Work out the finished part from the listing and answer in its coordinate system (mm). Coordinates: 2 decimals unless noted, no trailing zeros. Order: outer loops, then holes, each group sorted by start corner. A loop starts at its lowest first (then second) coordinate and runs counter-clockwise, first axis right, second up.
1. The part is cut by section A-A, the plane z = 85. Give the vertices of the cut face in (x, y).
2. The part is cut by section C-C, the plane x = 70. Give the vertices of the cut face in (y, z), then the cut area to 3 significant figures.
3. A flat-ended cylindrical pin translates along its axis: pin 1 Ø12.5 at (x, z) = (-45, 60) entering from +Y. Find the tip coordinate at first contact, or state that the pin passes through.
4. The part is cut by section D-D, the plane y = -3.5. Count the separate pieces of the cut face and the enclosed holes in it, then the cut area to 3 significant figures.
5. The part is cut by section B-B, the plane x = 0. Give the vertices of the cut face in (y, z), then the cut area to 3 significant figures.
6. Determine the mould class of faces 1 (the flat face through (-3, -5, 130)), 2 (the cylindrical face through (44.09, -4.93, 66.94)), 3 (the flat face through (180, -5, -2)), 4 (the flat face through (-180, -5, -2)) for opening direction X: +X half, -X half, draft (parallel to the pull), parting line (faces both ways), or undercut.
7. Find the intervals of material crossed by probe 1 along Z at (x, y) = (70, -3); probe 2 along X at (y, z) = (-1.25, -86); probe 3 along X at (y, z) = (-6.25, 81.5), in increasing order.
```python
from build123d import *

# Parameters (mm, degrees)
F0_W     = 360
F0_H     = 260
F0_R     = 20
F0_R_2   = 7
F0_R_3   = 47.5
F1_DEPTH = 10


with BuildPart() as f1:
    # F0 (on Front) → F1 (new body)
    with BuildSketch(Plane.XZ):
        Rectangle(F0_W, F0_H)
        with Locations((-70, -85)):
            Circle(F0_R, mode=Mode.SUBTRACT)
        with Locations((-45, -60)):
            Circle(F0_R_2, mode=Mode.SUBTRACT)
        with Locations((70, -85)):
            Circle(F0_R, mode=Mode.SUBTRACT)
        with Locations((45, -60)):
            Circle(F0_R_2, mode=Mode.SUBTRACT)
        with Locations((-45, 60)):
            Circle(F0_R_2, mode=Mode.SUBTRACT)
        with Locations((-70, 85)):
            Circle(F0_R, mode=Mode.SUBTRACT)
        Circle(F0_R_3, mode=Mode.SUBTRACT)
        with Locations((45, 60)):
            Circle(F0_R_2, mode=Mode.SUBTRACT)
        with Locations((70, 85)):
            Circle(F0_R, mode=Mode.SUBTRACT)
    extrude(amount=F1_DEPTH)


solid = f1.part
```
Geometry says:
1. outline: (-180, -10) - (-90, -10) - (-90, 0) - (-180, 0) - close; (-50, -10) - (50, -10) - (50, 0) - (-50, 0) - close; (90, -10) - (180, -10) - (180, 0) - (90, 0) - close
2. outline: (-10, -130) - (0, -130) - (0, -105) - (-10, -105) - close; (-10, -65) - (0, -65) - (0, 65) - (-10, 65) - close; (-10, 105) - (0, 105) - (0, 130) - (-10, 130) - close
2. area: 1,800 mm2
3. pin 1: passes through
4. separate pieces: 1
4. enclosed holes: 9
4. area: 80,900 mm2
5. outline: (-10, -130) - (0, -130) - (0, -47.5) - (-10, -47.5) - close; (-10, 47.5) - (0, 47.5) - (0, 130) - (-10, 130) - close
5. area: 1,650 mm2
6. face 1: draft
6. face 2: undercut
6. face 3: +X half
6. face 4: -X half
7. probe 1: z = -130 to -105, -65 to 65, 105 to 130
7. probe 2: x = -180 to -89.97, -50.03 to 50.03, 89.97 to 180
7. probe 3: x = -180 to -89.69, -50.31 to 50.31, 89.69 to 180
